The figure shows three views and two pictorial views of one solid part (mm, origin at its lowest corner). Answer the questions. A direction names the side the tool comes from. Round coordinates to 2 decimals unless told otherwise and drop trailing zeros. Order: outer loops, then holes, each group sorted by start corner. A loop starts at its lowest first (then second) coordinate and runs counter-clockwise, first axis right, second up. Notation, with made-up numbers: (24.5, 13.25) -> (50.5, 13.25) arc R23 cw to (50.5, 50.25) -> close; hole circle Ø7 at (45, 13.5). An arc over 180 degrees is marked (long way). One line per item, written item: value. Start each with the question number.
1. Consider line 1 (Y direction, x = 14.5, z = 15); line 2 (Z direction, x = 25.5, y = 28); line 3 (X direction, y = 146, z = 7). Determine where each line is inside the solid, lowest interval first.
2. For the marked faces 1, 2 and 3, determine the directions among +Z, -Z, +X, -X, +Y, -Y from which every point of the face is accessible in a straight line to the end or side of a thin tool.
3. Section A-A (y = 155) is taken. Give the vertices of the cut face in (x, z), then the cut area to 3 significant figures.
4. Section B-B (z = 16.5) is taken. Give the vertices of the cut face in (x, y), then the cut area to 3 significant figures.
5. Section D-D (y = 106) is taken. Give the vertices of the cut face in (x, z), then the cut area to 3 significant figures.
6. Section C-C (x = 7) is taken. Give the vertices of the cut face in (y, z).
7. Flat-ended cylindrical pins translate along their axes: pin 1 Ø6 at (x, z) = (17.5, 17) entering from +Y; pin 2 Ø3 at (x, z) = (16.5, 21) entering from -Y; pin 3 Ø10 at (x, y) = (17, 49) entering from -Z. Find the tip coordinate at first contact, or state that the pin passes through.
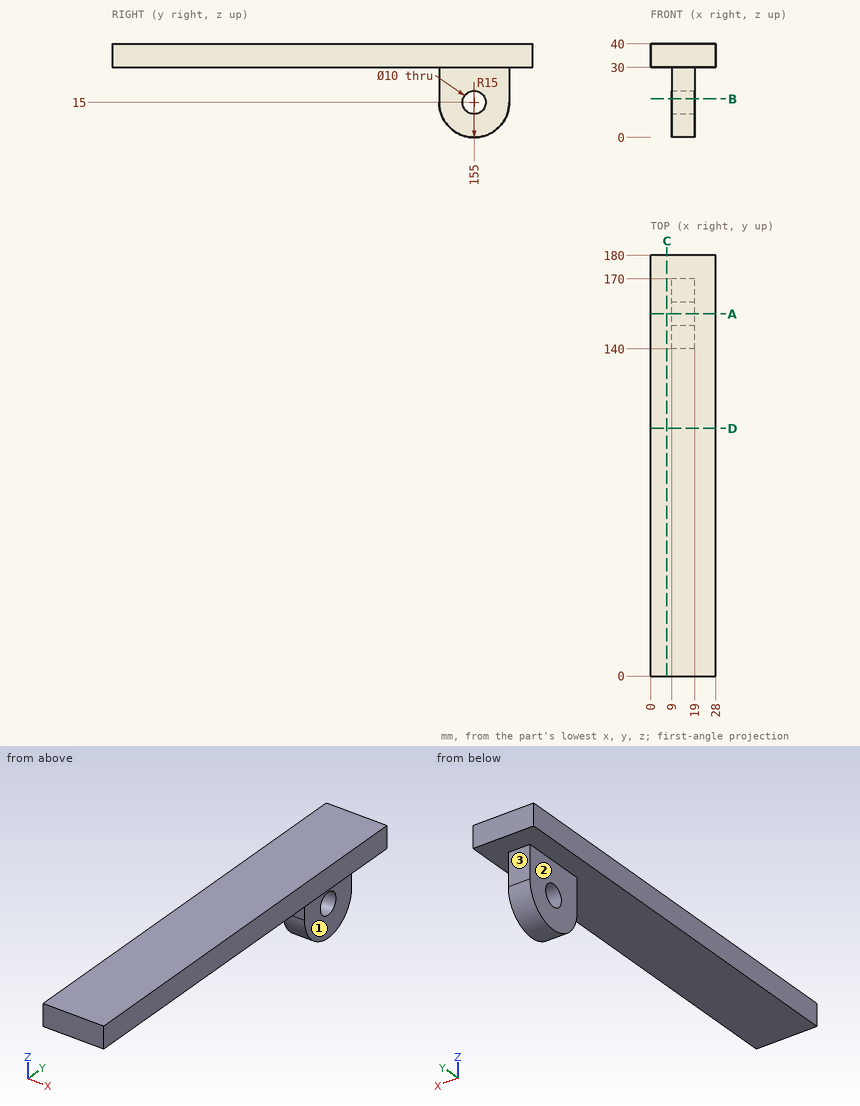
Answer:
1. line 1: 140 to 150, 160 to 170
1. line 2: 30 to 40
1. line 3: 9 to 19
2. face 1: -Z, +X, +Y, -Y
2. face 2: -Z, -X, +Y, -Y
2. face 3: -Z, +X, -X, +Y
3. outline: (0, 30) -> (9, 30) -> (9, 20) -> (19, 20) -> (19, 30) -> (28, 30) -> (28, 40) -> (0, 40) -> close; (9, 0) -> (19, 0) -> (19, 10) -> (9, 10) -> close
3. area: 480 mm^2
4. outline: (9, 140) -> (19, 140) -> (19, 150.23) -> (9, 150.23) -> close; (9, 159.77) -> (19, 159.77) -> (19, 170) -> (9, 170) -> close
4. area: 205 mm^2
5. outline: (0, 30) -> (28, 30) -> (28, 40) -> (0, 40) -> close
5. area: 280 mm^2
6. outline: (0, 30) -> (180, 30) -> (180, 40) -> (0, 40) -> close
7. pin 1: y = 170
7. pin 2: y = 140
7. pin 3: z = 30
